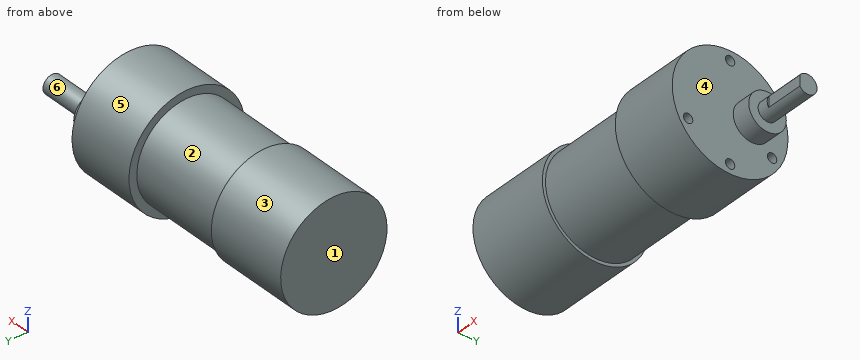
```python
from build123d import *

# Parameters (mm, degrees)
ESQUISSE2_R             = 6
BOSS_EXTRU_1_DEPTH      = 6
ESQUISSE3_R             = 3
BOSS_EXTRU_2_DEPTH      = 15.5
ESQUISSE4_W             = 12
ESQUISSE4_H             = 0.5
ENL_V_MAT_EXTRU_1_DEPTH = 7.75
ESQUISSE5_R             = 1.5
ENL_V_MAT_EXTRU_2_DEPTH = 3.5
ESQUISSE6_W             = 3
ESQUISSE6_H             = 1
BOSS_EXTRU_3_DEPTH      = 4
ESQUISSE7_R             = 17
BOSS_EXTRU_4_DEPTH      = 26.813317369


with BuildPart() as part:
    # Esquisse1 → Révolution1 (revolve)
    with BuildSketch(Plane.XY, mode=Mode.PRIVATE) as r_volution1_sk:
        Polygon((0, 0), (0, 2), (2, 2), (2, 16), (32, 16), (32, 18.5), (54, 18.5), (54, 0), align=None)
    revolve(r_volution1_sk.sketch.rotate(Axis((0, 0, 0), (1, 0, 0)), 90), axis=Axis((0, 0, 0), (1, 0, 0)))

    # Esquisse2 → Boss.-Extru.1 (add)
    with BuildSketch(Plane(origin=(54, 0, 0), x_dir=(0, 0, -1), z_dir=(1, 0, 0))):
        with Locations(Location((0, 7, 0), (0, 0, 180))):
            Circle(ESQUISSE2_R)
    extrude(amount=BOSS_EXTRU_1_DEPTH)

    # Esquisse3 → Boss.-Extru.2 (add)
    with BuildSketch(Plane(origin=(60, 0, 0), x_dir=(0, 0, -1), z_dir=(1, 0, 0))):
        with Locations((0, 7)):
            Circle(ESQUISSE3_R)
    extrude(amount=BOSS_EXTRU_2_DEPTH)

    # Esquisse4 → Enlèv. mat.-Extru.1 (cut, symmetric)
    with BuildSketch(Plane.XY):
        with Locations((69.5, 4.25)):
            Rectangle(ESQUISSE4_W, ESQUISSE4_H)
    extrude(amount=ENL_V_MAT_EXTRU_1_DEPTH, both=True, mode=Mode.SUBTRACT)

    # Esquisse5 → Enlèv. mat.-Extru.2 (cut)
    with BuildSketch(Plane(origin=(54, 0, 0), x_dir=(0, 0, -1), z_dir=(1, 0, 0))):
        with Locations((15.5, 0)):
            Circle(ESQUISSE5_R)
        with Locations((7.75, 13.423393759)):
            Circle(ESQUISSE5_R)
        with Locations((7.75, -13.423393759)):
            Circle(ESQUISSE5_R)
        with Locations((-15.5, 0)):
            Circle(ESQUISSE5_R)
    extrude(amount=-ENL_V_MAT_EXTRU_2_DEPTH, mode=Mode.SUBTRACT)

    # Esquisse6 → Boss.-Extru.3 (add)
    with BuildSketch(Plane.ZY.offset(-2)):
        with Locations((0, 12.939057981)):
            Rectangle(ESQUISSE6_W, ESQUISSE6_H)
        with Locations((0, -12.939057981)):
            Rectangle(ESQUISSE6_W, ESQUISSE6_H)
    extrude(amount=BOSS_EXTRU_3_DEPTH)

    # Esquisse7 → Boss.-Extru.4 (add)
    with BuildSketch(Plane.ZY.offset(-2)):
        Circle(ESQUISSE7_R)
    extrude(amount=BOSS_EXTRU_4_DEPTH)


solid = part.part
```
Geometry: final body of the model. Coordinates: model frame, mm. Face numbers are marked on the shaded views. A direction names the side the tool comes from. Coordinates: 2 decimals unless noted, no trailing zeros. Order: outer loops, then holes, each group sorted by start corner. A loop starts at its lowest first (then second) coordinate and runs counter-clockwise, first axis right, second up. Notation, with made-up numbers: (56, 16.5) - (86, 16.5) arc R9 ccw to (86, 21.5) - close; hole circle Ø1 at (19, 85.25). An arc over 180 degrees is marked (long way). Return JSON: item names as keys, results as strings. Group by question number.
1. Set-up query: the marked faces 5 and 6. Return all of +Z, -Z, +X, -X, +Y, -Y with unobstructed straight access to the full face (end or side cutting, diameter ignored); none if empty.
2. Cut plane A-A (z = 0). Output: boundary loops of the cut face in (x, y).
3. Material intervals for line 1 along Y through (x, z) = (51.3, -7.75); line 2 along X through (y, z) = (12.5, -11); line 3 along X through (y, z) = (-11, 6), sorted ascending. Write a range as [from, to].
4. Cut plane B-B (y = 0). Output: boundary loops of the cut face in (x, z).
5. Cut plane D-D (z = -7.75). Output: boundary loops of the cut face in (x, y).
6. Pull-direction query (X, two-part tool) for the marked faces 1, 2, 3 and 4; classes: pulls with the +X half, pulls with the -X half, needs draft (parallel to the pull), parting line crosses it, or undercut.
7. Pin query (flat end, axial travel): pin 1 (4 mm diameter, centred on y = 2.5, z = -3, fed in from +X); pin 2 (1.5 mm diameter, centred on y = 0.5, z = -15.5, fed in from +X); pin 3 (2.5 mm diameter, centred on y = -13, z = -7.5, fed in from +X); pin 4 (10 mm diameter, centred on x = 61, z = -11, fed in from -Y). Return the tip coordinate at first contact, or that it passes through.
8. Cut plane C-C (x = 27). Output: boundary loops of the cut face in (y, z), plus the area to 3 significant figures.
Resolved:
{
 "1": {"face 5": "+X, -X", "face 6": "+X"},
 "2": {"outline": "(-24.81, -17) - (2, -17) - (2, -16) - (32, -16) - (32, -18.5) - (54, -18.5) - (54, 1) - (60, 1) - (60, 4) - (63.5, 4) - (63.5, 4.5) - (75.5, 4.5) - (75.5, 10) - (60, 10) - (60, 13) - (54, 13) - (54, 18.5) - (32, 18.5) - (32, 16) - (2, 16) - (2, 17) - (-24.81, 17) - close"},
 "3": {"line 1": "y = [-16.8, -14.92], [-11.92, 11.92], [14.92, 16.8]", "line 2": "x = [-24.81, 2], [32, 54]", "line 3": "x = [-24.81, 54]"},
 "4": {"outline": "(-24.81, -17) - (2, -17) - (2, -16) - (32, -16) - (32, -18.5) - (54, -18.5) - (54, -17) - (50.5, -17) - (50.5, -14) - (54, -14) - (54, 14) - (50.5, 14) - (50.5, 17) - (54, 17) - (54, 18.5) - (32, 18.5) - (32, 16) - (2, 16) - (2, 17) - (-24.81, 17) - close"},
 "5": {"outline": "(-24.81, -15.13) - (2, -15.13) - (2, -14) - (32, -14) - (32, -16.8) - (54, -16.8) - (54, -14.92) - (50.5, -14.92) - (50.5, -11.92) - (54, -11.92) - (54, 11.92) - (50.5, 11.92) - (50.5, 14.92) - (54, 14.92) - (54, 16.8) - (32, 16.8) - (32, 14) - (2, 14) - (2, 15.13) - (-24.81, 15.13) - close"},
 "6": {"face 1": "pulls with the -X half", "face 2": "undercut", "face 3": "needs draft", "face 4": "pulls with the +X half"},
 "7": {"pin 1": "stops at x = 60", "pin 2": "stops at x = 50.5", "pin 3": "stops at x = 54", "pin 4": "passes through"},
 "8": {"outline": "circle Ø32 at (0, 0)", "area": "804 mm²"}
}
